```python
from build123d import *

# Parameters (mm, degrees)
BOSS_EXTRUDE1_DEPTH = 25.4
CUT_EXTRUDE1_REACH  = 53.18
SKETCH2_R           = 6.35
FILLET1_R           = 3.175
SKETCH3_R           = 7.14375
SKETCH3_R_2         = 6.35
BOSS_EXTRUDE2_DEPTH = 0.79375


with BuildPart() as part:
    # Sketch1 → Boss-Extrude1 (new body)
    with BuildSketch(Plane(origin=(0, 0, 0), x_dir=(0, 0, -1), z_dir=(1, 0, 0))):
        Polygon((2.54, 2.54), (25.4, 2.54), (25.4, 0), (0, 0), (0, 38.1), (2.54, 38.1), align=None)
    extrude(amount=BOSS_EXTRUDE1_DEPTH)

    # Sketch2 → Cut-Extrude1 (cut, up to next)
    with BuildSketch(Plane(origin=(0, 0, -2.54), x_dir=(-1, 0, 0), z_dir=(0, 0, -1)), mode=Mode.PRIVATE) as cut_extrude1_sk1:
        with Locations((-12.7, 30.1625)):
            Circle(SKETCH2_R)
    cut_extrude1_tool1 = extrude(cut_extrude1_sk1.sketch, amount=-CUT_EXTRUDE1_REACH, mode=Mode.PRIVATE) & part.part
    add(cut_extrude1_tool1.solids().sort_by_distance((12.7, 30.1625, -2.54))[0], mode=Mode.SUBTRACT)

    # Fillet1
    fillet1_edges = [part.edges().sort_by_distance(p)[0] for p in [
        (25.4, 38.1, -1.27),
        (0, 38.1, -1.27),
    ]]
    fillet(fillet1_edges, radius=FILLET1_R)

    # Sketch3 → Boss-Extrude2 (add)
    with BuildSketch(Plane.XY):
        with Locations(Location((12.7, 30.1625, 0), (0, 0, 180))):
            Circle(SKETCH3_R)
        with Locations(Location((12.7, 30.1625, 0), (0, 0, 180))):
            Circle(SKETCH3_R_2, mode=Mode.SUBTRACT)
    extrude(amount=BOSS_EXTRUDE2_DEPTH)


solid = part.part
```
Model file for the job. Use its own axes, mm. A direction names the side the tool comes from. Coordinates: 2 decimals unless noted, no trailing zeros. Order: outer loops, then holes, each group sorted by start corner. A loop starts at its lowest first (then second) coordinate and runs counter-clockwise, first axis right, second up. Notation, with made-up numbers: (-27, 50) - (24, 50) arc R10 ccw to (24, 68) - close; hole circle Ø7 at (-29, 44.25). An arc over 180 degrees is marked (long way). Return JSON: item names as keys, results as strings. Group by question number.
1) Saw through at D-D, the plane x = 4.25. Write the cut outline in (y, z), plus the area to 3 significant figures.
2) Saw through at C-C, the plane z = -10.75. Write the cut outline in (x, y), plus the area to 3 significant figures.
3) Saw through at B-B, the plane y = 10. Write the cut outline in (x, z), plus the area to 3 significant figures.
4) Probe line 1 (Y direction, x = 12.7, z = -1.45); line 2 (Y direction, x = 12, z = -17.75); line 3 (X direction, y = 30, z = -2). List the from-to ranges inside material, lowest first. Write a range as from..to.
5) Tool access for faces 1 (the flat face through (13, 21, -2.54)), 2 (the cylindrical face through (14.249, 37.136, 0.391)), 3 (the flat face through (25.4, 11, -2)): list every direction of +Z, -Z, +X, -X, +Y, -Y with a clear straight run to the whole face (end or side of a thin tool).
6) Saw through at A-A, the plane x = 12.7. Write the cut outline in (y, z), plus the area to 3 significant figures.
7) Flat gauge pins, fed straight in: P1, Ø4, axis at x = 19.5, z = -11, coming from the +Y side; P2, Ø12, axis at x = 7, y = 7, coming from the +Z side; P3, Ø6, axis at x = 6.5, y = 25.5, coming from the -Z side. Where does each tip first touch, or does it go through?
Values found:
{
 "1": {"outline": "(0, -25.4) - (2.54, -25.4) - (2.54, -2.54) - (38.1, -2.54) - (38.1, 0) - (0, 0) - close", "area": "155 mm²"},
 "2": {"outline": "(0, 0) - (25.4, 0) - (25.4, 2.54) - (0, 2.54) - close", "area": "64.5 mm²"},
 "3": {"outline": "(0, -2.54) - (25.4, -2.54) - (25.4, 0) - (0, 0) - close", "area": "64.5 mm²"},
 "4": {"line 1": "y = 0..23.81, 36.51..38.1", "line 2": "y = 0..2.54", "line 3": "x = 0..6.35, 19.05..25.4"},
 "5": {"face 1": "-Z, +X, -X, +Y", "face 2": "+Z", "face 3": "+Z, -Z, +X, +Y, -Y"},
 "6": {"outline": "(0, -25.4) - (2.54, -25.4) - (2.54, -2.54) - (23.81, -2.54) - (23.81, 0.79) - (23.02, 0.79) - (23.02, 0) - (0, 0) - close; (36.51, -2.54) - (38.1, -2.54) - (38.1, 0) - (37.31, 0) - (37.31, 0.79) - (36.51, 0.79) - close", "area": "124 mm²"},
 "7": {"P1": "stops at y = 2.54", "P2": "stops at z = 0", "P3": "stops at z = -2.54"}
}
